```python
from build123d import *

# Parameters (mm, degrees)
F1_DEPTH = 6.35
F3_DEPTH = 5.08
F6_D     = 6.35


with BuildPart() as f1:
    # F0 (on Front) → F1 (new body)
    with BuildSketch(Plane.XZ):
        with BuildLine():
            Line((-50.789758563, 12.7), (-50.8, 0))
            ThreePointArc((-50.8, 0), (-31.1513127772, -22.5475967725), (-3.5936811473, -10.9268408269))
            ThreePointArc((-3.5936811473, -10.9268408269), (0, -8.9034761257), (3.5936811473, -10.9268408269))
            ThreePointArc((3.5936811473, -10.9268408269), (31.1513127772, -22.5475967725), (50.8, 0))
            Line((50.8, 0), (50.789758563, 12.7))
            Line((50.789758563, 12.7), (0, 12.7))
            Line((0, 12.7), (-50.789758563, 12.7))
        make_face()
    extrude(amount=F1_DEPTH)

    # F2 (on face) → F3 (join)
    with BuildSketch(Plane(origin=(50.7999669647, 0, 0.0409657212), x_dir=(0, 1, 0), z_dir=(0.9999996748, 0, 0.0008064121))):
        with BuildLine():
            Line((46.1317837944, 12.6590383949), (0, 12.6590383949))
            Line((0, 12.6590383949), (0, 6.3090363302))
            Line((0, 6.3090363302), (43.3671333809, 6.3090363302))
            add(Edge.make_bspline(
                [(43.3671333809, 6.3090363302), (47.8048958927, 6.4029112237), (52.3956002369, 6.5378512338), (60.8254648697, -0.5707092536), (64.4781213146, -1.5761370426), (66.6516050696, -1.7843674764)],
                knots=[0, 0, 0, 0, 0.3549617082, 0.7163958478, 1, 1, 1, 1], degree=3))
            ThreePointArc((66.6516050696, -1.7843674764), (69.1195081439, 0.4583984006), (66.6516050696, 2.7011642776))
            add(Edge.make_bspline(
                [(46.1317837944, 12.6590383949), (49.0594556176, 12.5911172202), (50.0191314518, 12.0839436725), (60.2418071998, 4.8232645807), (65.3014332056, 2.1007801406), (66.6516050696, 2.7011642776)],
                knots=[0, 0, 0, 0, 0.2660253484, 0.6885067526, 1, 1, 1, 1], degree=3))
        make_face()
    extrude(amount=-F3_DEPTH)

    # F4: F1 across plane


with BuildPart() as f1_1:
    add(f1.part)
    add(f1.part.mirror(Plane.YZ))

    # F6 (through all)
    with Locations(Plane(origin=(0, 0, 0), x_dir=(1, 0, 0), z_dir=(0, 1, 0))):
        with Locations((25.4, -2.2993200155), (-25.4, -2.2993200155)):
            Hole(F6_D / 2)


solid = f1_1.part
```
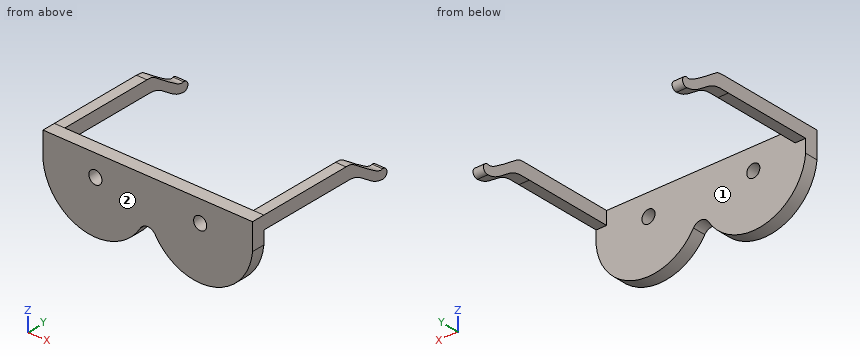
Can you work these out from the model? Positions are in its coordinate system, mm. Face numbers are marked on the shaded views. Coordinates: 2 decimals unless noted, no trailing zeros. Loops run counter-clockwise (first coordinate to the right, second up) from the corner with the lowest first, then second, coordinate; pieces in that order, holes last. Notation, with made-up numbers: (-29, 41) - (4, 41) arc R11 cw to (4, 52) - close; hole circle Ø11 at (50, -16). An arc over 180 degrees is marked (long way). Answer as CSV lines item,"result". Start each with the question number.
1) For pin 1 (8 mm diameter, centred on x = 37, z = 7.5, fed in from +Y); pin 2 (7.5 mm diameter, centred on x = -25.4, z = 2.3, fed in from -Y); pin 3 (3 mm diameter, centred on y = 58, z = 3.5, fed in from -X), each with a flat end and sliding along its axis, tell me the tip position at first contact or that it passes through.
2) Suppose I cut it at B-B (y = 6.5). Please give me the cut outline in (x, z), plus the area to 3 significant figures.
3) Suppose I cut it at D-D (x = -32). Please give me the cut outline in (y, z).
4) Thinking about a two-plate mould opening in X: for the marked faces 1 and 2, which applies, pulls with the +X half, pulls with the -X half, needs draft (parallel to the pull), parting line crosses it, or undercut?
5) Suppose I cut it at C-C (x = 44). Please give me the cut outline in (y, z).
6) Suppose I cut it at A-A (x = 25.4). Please give me the cut outline in (y, z), plus the area to 3 significant figures.
7) I need wall thicknesses on line 1 (Z direction, x = -25, y = -3); line 2 (X direction, y = 48, z = 7.5); line 3 (Z direction, x = -25.4, y = -3.25). Which ranges of each line are inside material? Lowest first, please. Write a range as from..to.
Check result:
1,pin 1,"stops at y = 0"
1,pin 2,"stops at y = -6.35"
1,pin 3,"stops at x = -50.8"
2,outline,"(-50.79, 6.35) - (-45.71, 6.35) - (-45.71, 12.7) - (-50.79, 12.7) - close; (45.71, 6.35) - (50.79, 6.35) - (50.79, 12.7) - (45.71, 12.7) - close"
2,area,"64.5 mm²"
3,outline,"(-6.35, -22.34) - (0, -22.34) - (0, 12.7) - (-6.35, 12.7) - close"
4,face 1,"undercut"
4,face 2,"needs draft"
5,outline,"(-6.35, -15.15) - (0, -15.15) - (0, 12.7) - (-6.35, 12.7) - close"
6,outline,"(-6.35, -23.2) - (0, -23.2) - (0, -0.88) - (-6.35, -0.88) - close; (-6.35, 5.47) - (0, 5.47) - (0, 12.7) - (-6.35, 12.7) - close"
6,area,"188 mm²"
7,line 1,"z = -23.2..-0.85, 5.45..12.7"
7,line 2,"x = -50.79..-45.71, 45.71..50.79"
7,line 3,"z = -23.2..-0.88, 5.47..12.7"
